Job drawing, mm, ordinate dimensions from the low corner. One solid piece. Give positions to 0.01 mm unless a question says otherwise; leave off trailing zeros. Order: outer loops, then holes, each group sorted by start corner. A loop starts at its lowest first (then second) coordinate and runs counter-clockwise, first axis right, second up. Notation, with made-up numbers: (10, 32) - (58, 32) arc R14 cw to (58, 38) - close; hole circle Ø8 at (5, 50). An arc over 180 degrees is marked (long way). One line per item, written item: value.
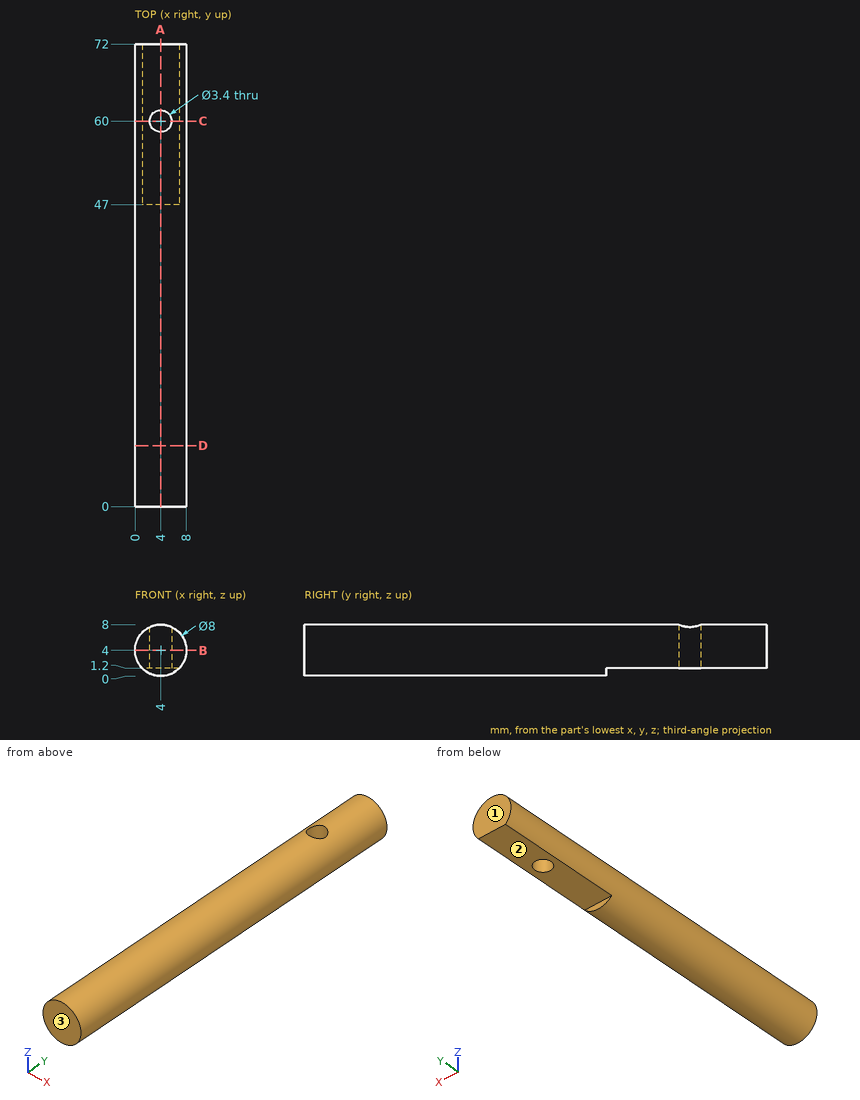
1) Wall check: line 1 along Y through (x, z) = (4, 4.25); line 2 along Z through (x, y) = (4.25, 30.5); line 3 along Y through (x, z) = (3, 0.5). Give the ranges that are in metal, low to high. Write a range as [from, to].
Answer:
line 1: y = [0, 58.3], [61.7, 72]
line 2: z = [0.01, 7.99]
line 3: y = [0, 47]
2) Slice it at D-D on y = 9.5. Write the cut outline in (x, z), then the cut area to 3 significant figures.
Answer:
outline: circle Ø8 at (4, 4)
area: 50.3 mm2
3) Slice it at C-C on y = 60. Write the cut outline in (x, z), then the cut area to 3 significant figures.
Answer:
outline: (1.14, 1.2) - (2.3, 1.2) - (2.3, 7.62) arc R4 ccw to start; (5.7, 1.2) - (6.86, 1.2) arc R4 ccw to (5.7, 7.62) - close
area: 22.8 mm2
4) Slice it at A-A on x = 4. Write the cut outline in (y, z).
Answer:
outline: (0, 0) - (47, 0) - (47, 1.2) - (58.3, 1.2) - (58.3, 8) - (0, 8) - close; (61.7, 1.2) - (72, 1.2) - (72, 8) - (61.7, 8) - close
5) Two-plate mould, pull along Y, no slides. Class the marked faces 1, 2 and 3: pulls with the +Y half, pulls with the -Y half, needs draft (parallel to the pull), parting line crosses it, or undercut.
Answer:
face 1: pulls with the +Y half
face 2: needs draft
face 3: pulls with the -Y half
6) Slice it at B-B on z = 4. Write the cut outline in (x, y).
Answer:
outline: (0, 0) - (8, 0) - (8, 72) - (0, 72) - close; hole circle Ø3.4 at (4, 60)
7) Drop flat-ended pins along their axis: P1, Ø1.5, axis at y = 27, z = 2, coming from the -X side; P2, Ø4.5, axis at x = 5, y = 58, coming from the -Z side; P3, Ø1, axis at x = 4.5, z = 0.5, coming from the +Y side; P4, Ø4, axis at x = 5, y = 37, coming from the +Z side. Give the stop position or say it passes through.
Answer:
P1: stops at x = 0.2
P2: stops at z = 1.2
P3: stops at y = 47
P4: stops at z = 8
